The listing builds one solid part. Answer for the finished solid, in the listing's coordinates (mm). Face numbers are marked on the shaded views. A direction names the side the tool comes from. Coordinates: 2 decimals unless noted, no trailing zeros. Write each loop counter-clockwise with the first axis right and the second up, starting at its lowest first coordinate (ties: lowest second). Pieces come first, ordered by that corner, then holes.
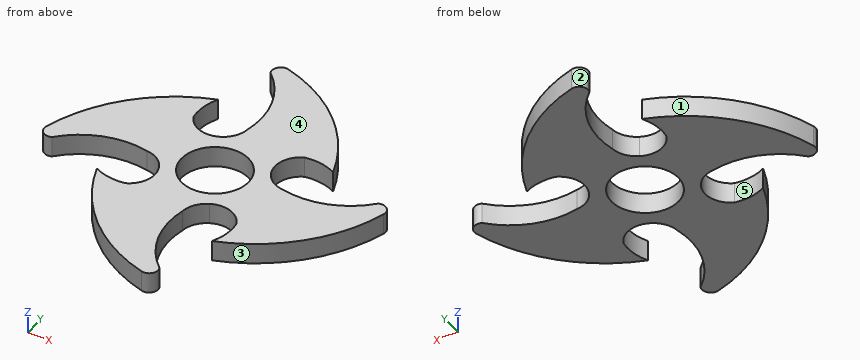
from build123d import *

# Parameters (mm, degrees)
F0_R        = 11.3
F1_DEPTH    = 7
F2_T1_DEPTH = 55.4992808982


# Not quite as in the source:
# - a fillet or chamfer that OpenCascade refuses, or shapes differently, is made with other operations: its cross-section is extruded or revolved along the edge and cut away or added
# - a feature names something its author has since deleted; it is built from what else it names


with BuildPart() as f1:
    # F0 (on Top) → F1 (new body)
    with BuildSketch(Plane.XY):
        with BuildLine():
            ThreePointArc((-19.0188516855, 18.6660698042), (-19.106601179, 24.2218879742), (-17.3798078978, 29.5032704141))
            ThreePointArc((-17.3798078978, 29.5032704141), (-42.8794362662, 11.5553714496), (-54.5032704141, -17.3798078978))
            ThreePointArc((-54.5032704141, -17.3798078978), (-51.6509498036, -14.2819027835), (-48.6055213036, -11.3736190606))
            ThreePointArc((-48.6055213036, -11.3736190606), (-36.3546417903, -3.2999675651), (-21.7060170396, -2.4719034169))
            ThreePointArc((-21.7060170396, -2.4719034169), (-17.5157178103, -3.9318400494), (-14.5899419176, -7.2679842351))
            ThreePointArc((-14.5899419176, -7.2679842351), (-15.4558877949, 5.1774059597), (-7.2679841768, 14.5899419466))
            ThreePointArc((-7.2679841768, 14.5899419466), (-14.000366861, 14.1575501664), (-19.0188516855, 18.6660698042))
        make_face()
        with BuildLine():
            ThreePointArc((-2.4719034169, 21.7060170396), (-3.9318400312, 17.5157178373), (-7.2679841768, 14.5899419466))
            ThreePointArc((-7.2679841768, 14.5899419466), (5.177405829, 15.4558878387), (14.5899417947, 7.2679844819))
            ThreePointArc((14.5899417947, 7.2679844819), (14.1575502222, 14.000367022), (18.6660698042, 19.0188516855))
            ThreePointArc((18.6660698042, 19.0188516855), (24.2218879742, 19.106601179), (29.5032704141, 17.3798078978))
            ThreePointArc((29.5032704141, 17.3798078978), (11.5553714496, 42.8794362662), (-17.3798078978, 54.5032704141))
            ThreePointArc((-17.3798078978, 54.5032704141), (-14.2819027835, 51.6509498036), (-11.3736190606, 48.6055213036))
            ThreePointArc((-11.3736190606, 48.6055213036), (-3.2999675651, 36.3546417903), (-2.4719034169, 21.7060170396))
        make_face()
        with BuildLine():
            ThreePointArc((14.5899417947, 7.2679844819), (5.177405829, 15.4558878387), (-7.2679841768, 14.5899419466))
            ThreePointArc((-7.2679841768, 14.5899419466), (-15.4558877949, 5.1774059597), (-14.5899419176, -7.2679842351))
            ThreePointArc((-14.5899419176, -7.2679842351), (-5.1774060707, -15.4558877577), (7.2679839673, -14.589942051))
            ThreePointArc((7.2679839673, -14.589942051), (13.8592593357, -8.5796812684), (16.3, 0))
            ThreePointArc((16.3, 0), (15.8667269979, 3.733225733), (14.5899417947, 7.2679844819))
        make_face()
        Circle(F0_R, mode=Mode.SUBTRACT)
        with BuildLine():
            ThreePointArc((7.2679839673, -14.589942051), (-5.1774060707, -15.4558877577), (-14.5899419176, -7.2679842351))
            ThreePointArc((-14.5899419176, -7.2679842351), (-14.157550177, -14.0003668918), (-18.6660698042, -19.0188516855))
            ThreePointArc((-18.6660698042, -19.0188516855), (-24.2218879742, -19.106601179), (-29.5032704141, -17.3798078978))
            ThreePointArc((-29.5032704141, -17.3798078978), (-11.5553714496, -42.8794362662), (17.3798078978, -54.5032704141))
            ThreePointArc((17.3798078978, -54.5032704141), (14.2819027835, -51.6509498036), (11.3736190606, -48.6055213036))
            ThreePointArc((11.3736190606, -48.6055213036), (3.2999675651, -36.3546417903), (2.4719034169, -21.7060170396))
            ThreePointArc((2.4719034169, -21.7060170396), (3.9318399658, -17.5157179344), (7.2679839673, -14.589942051))
        make_face()
        with BuildLine():
            ThreePointArc((21.7060170396, 2.4719034169), (17.515717696, 3.9318401265), (14.5899417947, 7.2679844819))
            ThreePointArc((14.5899417947, 7.2679844819), (15.8667269979, 3.733225733), (16.3, 0))
            ThreePointArc((16.3, 0), (13.8592593357, -8.5796812684), (7.2679839673, -14.589942051))
            ThreePointArc((7.2679839673, -14.589942051), (14.0003667504, -14.157550128), (19.0188516855, -18.6660698042))
            ThreePointArc((19.0188516855, -18.6660698042), (19.106601179, -24.2218879742), (17.3798078978, -29.5032704141))
            ThreePointArc((17.3798078978, -29.5032704141), (42.8794362662, -11.5553714496), (54.5032704141, 17.3798078978))
            ThreePointArc((54.5032704141, 17.3798078978), (51.6509498036, 14.2819027835), (48.6055213036, 11.3736190606))
            ThreePointArc((48.6055213036, 11.3736190606), (36.3546417903, 3.2999675651), (21.7060170396, 2.4719034169))
        make_face()
    extrude(amount=F1_DEPTH)

    # F2: fillet of radius 3 on 4 edges, made by hand

    # F2_s2 → F2_t1 (cut)
    with BuildSketch(Plane.XY.offset(-24.2496404491)):
        with BuildLine():
            ThreePointArc((-52.7416075724, -7.8412674467), (-51.7993975119, -10.9256989731), (-48.6055213036, -11.3736190606))
            ThreePointArc((-48.6055213036, -11.3736190606), (-51.6509498036, -14.2819027835), (-54.5032704141, -17.3798078978))
            ThreePointArc((-54.5032704141, -17.3798078978), (-53.8333652751, -12.5715819227), (-52.7416075724, -7.8412674467))
        make_face()
        with BuildLine():
            ThreePointArc((7.8412674467, -52.7416075724), (10.9256989731, -51.7993975119), (11.3736190606, -48.6055213036))
            ThreePointArc((11.3736190606, -48.6055213036), (14.2819027835, -51.6509498036), (17.3798078978, -54.5032704141))
            ThreePointArc((17.3798078978, -54.5032704141), (12.5715819227, -53.8333652751), (7.8412674467, -52.7416075724))
        make_face()
        with BuildLine():
            ThreePointArc((52.7416075724, 7.8412674467), (51.7993975119, 10.9256989731), (48.6055213036, 11.3736190606))
            ThreePointArc((48.6055213036, 11.3736190606), (51.6509498036, 14.2819027835), (54.5032704141, 17.3798078978))
            ThreePointArc((54.5032704141, 17.3798078978), (53.8333652751, 12.5715819227), (52.7416075724, 7.8412674467))
        make_face()
        with BuildLine():
            ThreePointArc((-7.8412674467, 52.7416075724), (-10.9256989731, 51.7993975119), (-11.3736190606, 48.6055213036))
            ThreePointArc((-11.3736190606, 48.6055213036), (-14.2819027835, 51.6509498036), (-17.3798078978, 54.5032704141))
            ThreePointArc((-17.3798078978, 54.5032704141), (-12.5715819227, 53.8333652751), (-7.8412674467, 52.7416075724))
        make_face()
    extrude(amount=F2_T1_DEPTH, mode=Mode.SUBTRACT)


solid = f1.part
Q1. The part is cut by section C-C, the plane z = 5.5. Write down the section's boundary in (x, y).
Answers below:
outline: (-52.74, -7.84) arc R3 ccw to (-48.61, -11.37) arc R28.21 cw to (-21.71, -2.47) arc R8.7 cw to (-18.67, -19.02) arc R16.82 cw to (-29.5, -17.38) arc R54.94 ccw to (7.84, -52.74) arc R3 ccw to (11.37, -48.61) arc R28.21 cw to (2.47, -21.71) arc R8.7 cw to (19.02, -18.67) arc R16.82 cw to (17.38, -29.5) arc R54.94 ccw to (52.74, 7.84) arc R3 ccw to (48.61, 11.37) arc R28.21 cw to (21.71, 2.47) arc R8.7 cw to (18.67, 19.02) arc R16.82 cw to (29.5, 17.38) arc R54.94 ccw to (-7.84, 52.74) arc R3 ccw to (-11.37, 48.61) arc R28.21 cw to (-2.47, 21.71) arc R8.7 cw to (-19.02, 18.67) arc R16.82 cw to (-17.38, 29.5) arc R54.94 ccw to start; hole circle Ø22.6 at (0, 0)
Q2. The part is cut by section D-D, the plane x = 25. Write down the section's boundary in (y, z), then the cut area to 3 significant figures.
Answers below:
outline: (-26.27, 0) - (1.98, 0) - (1.98, 7) - (-26.27, 7) - close; (18.97, 0) - (27.33, 0) - (27.33, 7) - (18.97, 7) - close
area: 256 mm2
Q3. Find the intervals of material crossed by probe 1 along Y at (x, z) = (-4.5, 4); probe 2 along X at (y, z) = (-23.5, 2); probe 3 along Y at (x, z) = (15, 5.5), in increasing order.
Answers below:
probe 1: y = -47.63 to -10.37, 10.37 to 16.76, 39.38 to 51.7
probe 2: x = -27.02 to 2.16, 19.2 to 29.77
probe 3: y = -14.58 to 6.54, 15.76 to 39.91
Q4. The part is cut by section A-A, the plane x = -6. Write down the section's boundary in (y, z).
Answers below:
outline: (-46.75, 0) - (-9.58, 0) - (-9.58, 7) - (-46.75, 7) - close; (9.58, 0) - (15.36, 0) - (15.36, 7) - (9.58, 7) - close; (42.18, 0) - (52.2, 0) - (52.2, 7) - (42.18, 7) - close
Q5. Given pin 1 (20.5 mm diameter, centred on x = 0, y = 0, fed in from -Z); pin 2 (4 mm diameter, centred on x = -17.5, z = 5.5, fed in from +Y), each flat-ended and moving along its own axis, determine where each tip first touches the part or whether it passes through.
Answers below:
pin 1: passes through
pin 2: stops at y = 29.5
Q6. The part is cut by section B-B, the plane y = 0. Write down the section's boundary in (x, z), then the cut area to 3 significant figures.
Answers below:
outline: (-49.91, 0) - (-11.3, 0) - (-11.3, 7) - (-49.91, 7) - close; (11.3, 0) - (49.91, 0) - (49.91, 7) - (11.3, 7) - close
area: 540 mm2
Q7. Which of the six approach directions +Z, -Z, +X, -X, +Y, -Y give full straight-line access (tool end or side, diameter ignored) to the marked faces 4 and 5?
Answers below:
face 4: +Z, +X, -X, +Y, -Y
face 5: +Z, -Z
Q8. Determine the mould class of the marked faces 1, 2 and 3 for opening direction Y: released by +Y, released by -Y, zero draft, split by the parting line, or undercut.
Answers below:
face 1: released by +Y
face 2: undercut
face 3: released by -Y
